```python
from build123d import *

# Parameters (mm, degrees)
SALIENTE_EXTRUIR1_DEPTH = 2.5
CROQUIS2_R              = 1.5
CORTAR_EXTRUIR2_DEPTH   = 2.5


with BuildPart() as part:
    # Croquis1 → Saliente-Extruir1 (new body)
    with BuildSketch(Plane.XY):
        Polygon((-35.040719462, 0), (-35.040719462, 2.5), (-31.040719462, 4.25), (-27.040719462, 2.5), (-27.040719462, -2.5), (-31.040719462, -4.25), (-35.040719462, -2.5), align=None)
    extrude(amount=SALIENTE_EXTRUIR1_DEPTH)

    # Croquis2 → Cortar-Extruir2 (cut)
    with BuildSketch(Plane.XY.offset(2.5)):
        with Locations((-31.040719462, 0)):
            Circle(CROQUIS2_R)
    extrude(amount=-CORTAR_EXTRUIR2_DEPTH, mode=Mode.SUBTRACT)


solid = part.part
```
Verification items for the finished model (mm, model axes). Give positions to 0.01 mm unless a question says otherwise; leave off trailing zeros. Order: outer loops, then holes, each group sorted by start corner. A loop starts at its lowest first (then second) coordinate and runs counter-clockwise, first axis right, second up. Notation, with made-up numbers: (-14.75, -38) -> (32.25, -38) arc R31 ccw to (32.25, -6) -> close; hole circle Ø10 at (-34, 39.25). An arc over 180 degrees is marked (long way). One line per item, written item: value.
(1) Sectioned sample at C-C on x = -31.5. Record the cut outline in (y, z).
Final values:
outline: (-4.05, 0) -> (-1.43, 0) -> (-1.43, 2.5) -> (-4.05, 2.5) -> close; (1.43, 0) -> (4.05, 0) -> (4.05, 2.5) -> (1.43, 2.5) -> close
(2) Sectioned sample at A-A on y = 0. Record the cut outline in (x, z), then the cut area to 3 significant figures.
Final values:
outline: (-35.04, 0) -> (-32.54, 0) -> (-32.54, 2.5) -> (-35.04, 2.5) -> close; (-29.54, 0) -> (-27.04, 0) -> (-27.04, 2.5) -> (-29.54, 2.5) -> close
area: 12.5 mm^2
(3) Scan lines: line 1 along Y through (x, z) = (-31.5, 2.05); line 2 along Y through (x, z) = (-32, 0.4); line 3 along X through (y, z) = (-0.5, 1.95). Record each from-to range of solid material in increasing order. Write a range as [from, to].
Final values:
line 1: [-4.05, -1.43], [1.43, 4.05]
line 2: [-3.83, -1.15], [1.15, 3.83]
line 3: [-35.04, -32.45], [-29.63, -27.04]
(4) Sectioned sample at D-D on y = 2.75. Record the cut outline in (x, z).
Final values:
outline: (-34.47, 0) -> (-27.61, 0) -> (-27.61, 2.5) -> (-34.47, 2.5) -> close
(5) Gauge pin test, flat end, axial feed: pin 1 (1 mm diameter, centred on x = -33, z = 0.5, fed in from -Y). Record the tip position at first contact, or that the pin passes through.
Final values:
pin 1: y = -3.61
(6) Sectioned sample at B-B on z = 0.75. Record the cut outline in (x, y), then the cut area to 3 significant figures.
Final values:
outline: (-35.04, -2.5) -> (-31.04, -4.25) -> (-27.04, -2.5) -> (-27.04, 2.5) -> (-31.04, 4.25) -> (-35.04, 2.5) -> close; hole circle Ø3 at (-31.04, 0)
area: 46.9 mm^2
(7) Draft check along X on faces 1 (the face through (-29.01, -3.36, 1.23)), 2 (the face through (-33.069, 3.363, 1.232)), 3 (the face through (-29.61, 0.45, 1.27)). Enter one of: pulls with the +X half, pulls with the -X half, needs draft (parallel to the pull), parting line crosses it, or undercut.
Final values:
face 1: pulls with the +X half
face 2: pulls with the -X half
face 3: undercut
